Read the model definition and answer for the solid it produces. Units are mm, in the model's axes. Face numbers are marked on the shaded views. Coordinates: 2 decimals unless noted, no trailing zeros. Loops run counter-clockwise (first coordinate to the right, second up) from the corner with the lowest first, then second, coordinate; pieces in that order, holes last. Notation, with made-up numbers: (51.5, -31.75) - (105.5, -31.75) arc R17 ccw to (105.5, -23.75) - close; hole circle Ø1 at (-12.5, -15.75). An arc over 180 degrees is marked (long way). Use one line per item in the form item = value.
from build123d import *

# Parameters (mm, degrees)
F0_W     = 177.8
F0_H     = 127
F1_DEPTH = 50.8
F2_R     = 25.4
F3_DEPTH = 101.601
F4_R     = 9.525


with BuildPart() as f1:
    # F0 (on Top) → F1 (new body, symmetric)
    with BuildSketch(Plane.XY):
        Rectangle(F0_W, F0_H)
    extrude(amount=F1_DEPTH, both=True)

    # F2 (on face) → F3 (cut, through all)
    with BuildSketch(Plane.XY.offset(50.8)):
        Circle(F2_R)
    extrude(amount=-F3_DEPTH, mode=Mode.SUBTRACT)

    # F4
    f4_edges = [f1.edges().sort_by_distance(p)[0] for p in [
        (0, -63.5, 50.8),
        (-88.9, 0, 50.8),
        (88.9, 0, 50.8),
        (0, 63.5, 50.8),
    ]]
    fillet(f4_edges, radius=F4_R)


solid = f1.part
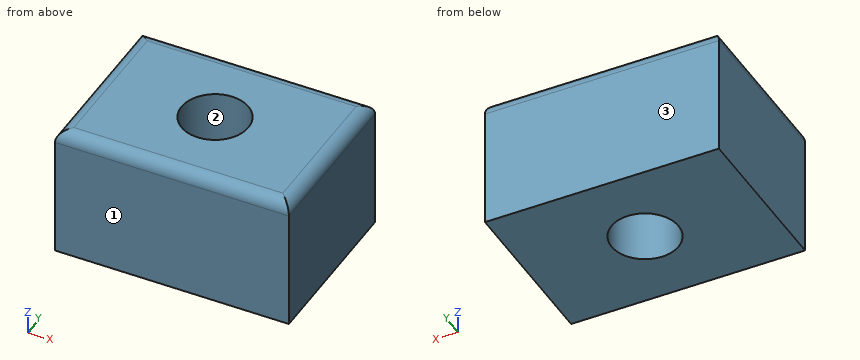
Item 1: The part is cut by section A-A on y = 0. Give the vertices of the cut face in (x, z) (3 decimals), plus the area to 3 significant figures.
Results below:
outline = (-88.9, -50.8) - (-25.4, -50.8) - (-25.4, 50.8) - (-79.375, 50.8) arc R9.525 ccw to (-88.9, 41.275) - close; (25.4, -50.8) - (88.9, -50.8) - (88.9, 41.275) arc R9.525 ccw to (79.375, 50.8) - (25.4, 50.8) - close
area = 12,900 mm²
Item 2: For a pull along Y with two mould halves and no side action, classify the marked faces 1, 2 and 3 as +Y half, -Y half, draft (parallel to the pull), parting line (faces both ways), or undercut.
Results below:
face_1 = -Y half
face_2 = undercut
face_3 = +Y half
Item 3: The part is cut by section B-B on x = 0. Give the vertices of the cut face in (y, z) (3 decimals).
Results below:
outline = (-63.5, -50.8) - (-25.4, -50.8) - (-25.4, 50.8) - (-53.975, 50.8) arc R9.525 ccw to (-63.5, 41.275) - close; (25.4, -50.8) - (63.5, -50.8) - (63.5, 41.275) arc R9.525 ccw to (53.975, 50.8) - (25.4, 50.8) - close
Item 4: The part is cut by section C-C on z = 2.5. Give the vertices of the cut face in (x, y).
Results below:
outline = (-88.9, -63.5) - (88.9, -63.5) - (88.9, 63.5) - (-88.9, 63.5) - close; hole circle Ø50.8 at (0, 0)
Item 5: Find the intervals of material crossed by L1, parallel to Y at x = 0, z = -6; L2, parallel to X at y = 18, z = -32; L3, parallel to Y at x = 23, z = -6, in increasing order.
Results below:
L1 = -63.5 to -25.4, 25.4 to 63.5
L2 = -88.9 to -17.92, 17.92 to 88.9
L3 = -63.5 to -10.78, 10.78 to 63.5
